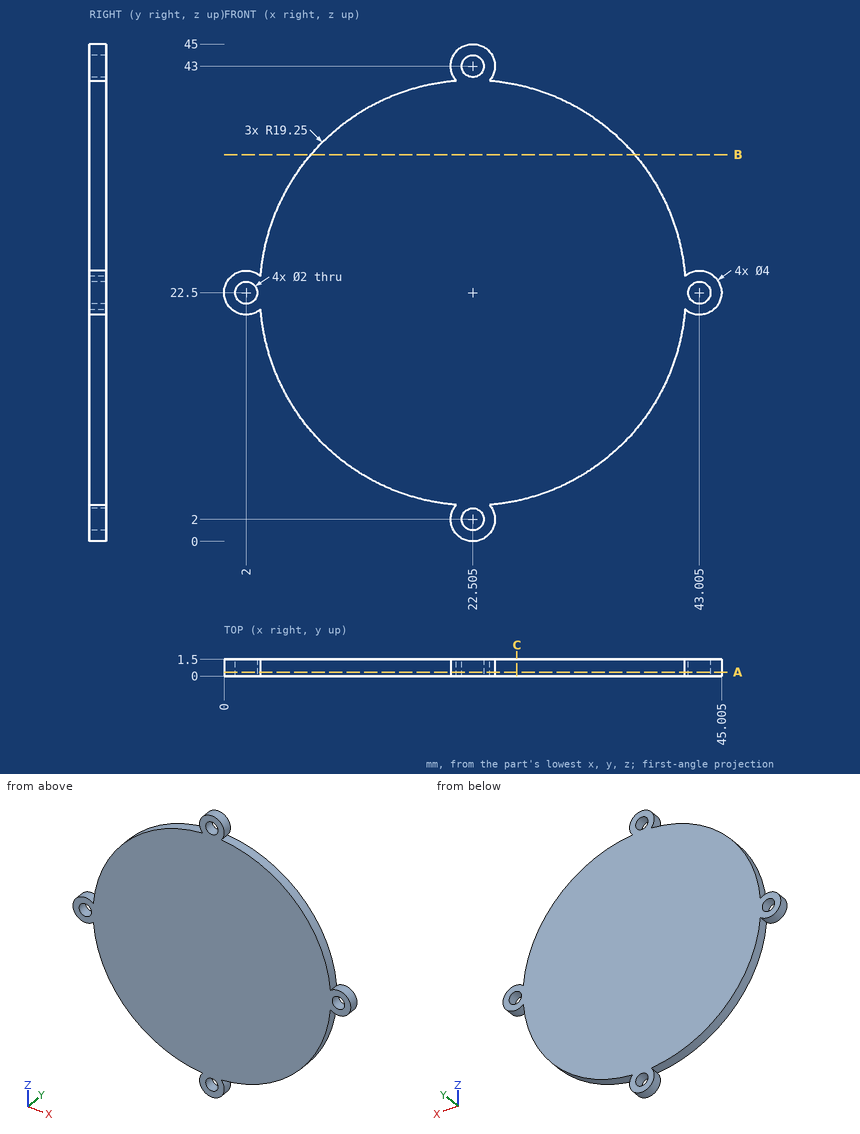
Could you check a few things on this drawing? It's one solid part, dimensions in mm from its lowest x, y, z. Round coordinates to 2 decimals unless told otherwise and drop trailing zeros. Order: outer loops, then holes, each group sorted by start corner. A loop starts at its lowest first (then second) coordinate and runs counter-clockwise, first axis right, second up. Notation, with made-up numbers: M 11.25,-21.75 L 50.25,-21.75 A26 ccw 50.25,17.25 Z; hole C 25.25,20 d10. An arc over 180 degrees is marked long. One line per item, written item: value.
(1) Imagine slicing it at A-A (y = 0.35). Count the separate pieces of the cut face and the enclosed holes in it, and give its area (3 significant figures).
Ans:
separate pieces: 1
enclosed holes: 4
area: 1,200 mm^2
(2) Imagine slicing it at B-B (z = 35). Write out the boundary of the cut face in (x, y), and give its area (3 significant figures).
Ans:
outline: M 7.87,0 L 37.14,0 L 37.14,1.5 L 7.87,1.5 Z
area: 43.9 mm^2
(3) I'm going to push a flat-ended pin straight in: P1, Ø1.6, axis at x = 2, z = 22.5, coming from the -Y side. Where does the tip first touch, or does it pass through?
Ans:
P1: passes through
(4) Imagine slicing it at C-C (x = 26.5). Write out the boundary of the cut face in (y, z).
Ans:
outline: M 0,3.67 L 1.5,3.67 L 1.5,41.33 L 0,41.33 Z
(5) I need wall thicknesses on line 1 along Z through (x, y) = (23, 1.2); line 2 along X through (y, z) = (0.6, 22) (1 decimal); line 3 along X through (y, z) = (1.35, 14.5). Which ranges of each line are inside material? Lowest first, please. Write a range as from..to.
Ans:
line 1: z = 0.06..1.13, 2.87..42.13, 43.87..44.94
line 2: x = 0.1..1.1, 2.9..42.1, 43.9..44.9
line 3: x = 5..40.01
